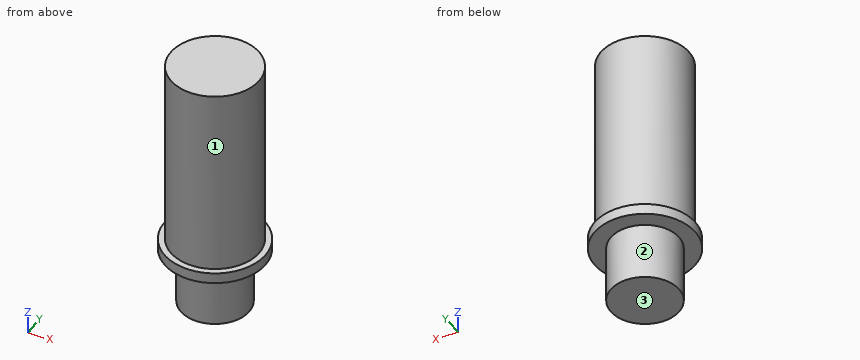
from build123d import *

# Parameters (mm, degrees)
F0_R     = 2.413
F1_DEPTH = 4.064
F2_R     = 3.556
F2_R_2   = 2.413
F3_DEPTH = 0.762
F4_R     = 3.1115
F5_DEPTH = 13.462


with BuildPart() as f1:
    # F0 (on Top) → F1 (new body)
    with BuildSketch(Plane.XY):
        with Locations((-47.52272, 37.3201)):
            Circle(F0_R)
    extrude(amount=F1_DEPTH)

    # F2 (on face) → F3 (join)
    with BuildSketch(Plane.XY.offset(4.064)):
        with Locations((-47.52272, 37.3201)):
            Circle(F2_R)
        with Locations((-47.52272, 37.3201)):
            Circle(F2_R_2, mode=Mode.SUBTRACT)
        with Locations((-47.52272, 37.3201)):
            Circle(F2_R_2)
    extrude(amount=F3_DEPTH)

    # F4 (on face) → F5 (join)
    with BuildSketch(Plane.XY.offset(4.826)):
        with Locations((-47.52272, 37.3201)):
            Circle(F4_R)
    extrude(amount=F5_DEPTH)


solid = f1.part
Here's how the part is built. I have some questions about the finished solid (model axes, mm). Face numbers are marked on the shaded views. A direction names the side the tool comes from. Round coordinates to 2 decimals unless told otherwise and drop trailing zeros. Loops run counter-clockwise (first coordinate to the right, second up) from the corner with the lowest first, then second, coordinate; pieces in that order, holes last. Notation, with made-up numbers: (-17.5, 43) - (-4.5, 43) arc R25 ccw to (-4.5, 80) - close; hole circle Ø2 at (47, 28). An arc over 180 degrees is marked (long way). One line per question, with ' | ' between items. Start each with the question number.
Q1. I want a section at D-D (y = 40). Write out the boundary of the cut face in (x, z).
Q2. For the marked faces 1, 2 and 3, which set-ups out of +Z, -Z, +X, -X, +Y, -Y let a thin tool reach every point of the face, with its end or its side?
Q3. I want a section at A-A (x = -45.5). Write out the boundary of the cut face in (y, z).
Q4. Please list where these lines run through material, in increasing order: line 1 (Z direction, x = -44.75, y = 39); line 2 (Z direction, x = -50, y = 36.75); line 3 (X direction, y = 37.5, z = 6.75). Write a range as [from, to].
Q5. I want a section at C-C (z = 7). Write out the boundary of the cut face in (x, y), then the cut area to 3 significant figures.
Q6. Will these pins go through, and if not, where does the flat tip stop? pin 1 (1.5 mm diameter, centred on y = 39.5, z = 8.5, fed in from +X); pin 2 (1 mm diameter, centred on x = -45.5, y = 35, fed in from -Z); pin 3 (4 mm diameter, centred on y = 35.5, z = 8.5, fed in from +X).
Q7. I want a section at B-B (y = 36). Write out the boundary of the cut face in (x, z), then the cut area to 3 significant figures.
Response values:
1) outline: (-49.86, 4.06) - (-45.19, 4.06) - (-45.19, 4.83) - (-45.94, 4.83) - (-45.94, 18.29) - (-49.1, 18.29) - (-49.1, 4.83) - (-49.86, 4.83) - close
2) face 1: +Z | face 2: -Z | face 3: -Z, +X, -X, +Y, -Y
3) outline: (34.4, 4.06) - (36, 4.06) - (36, 0) - (38.64, 0) - (38.64, 4.06) - (40.24, 4.06) - (40.24, 4.83) - (39.68, 4.83) - (39.68, 18.29) - (34.96, 18.29) - (34.96, 4.83) - (34.4, 4.83) - close
4) line 1: z = [4.06, 4.83] | line 2: z = [4.06, 18.29] | line 3: x = [-50.63, -44.42]
5) outline: circle Ø6.22 at (-47.52, 37.32) | area: 30.4 mm²
6) pin 1: stops at x = -44.76 | pin 2: stops at z = 4.06 | pin 3: stops at x = -44.41
7) outline: (-50.82, 4.06) - (-49.54, 4.06) - (-49.54, 0) - (-45.5, 0) - (-45.5, 4.06) - (-44.22, 4.06) - (-44.22, 4.83) - (-44.71, 4.83) - (-44.71, 18.29) - (-50.34, 18.29) - (-50.34, 4.83) - (-50.82, 4.83) - close | area: 97.3 mm²
